Check sheet for the modelled part. Datum: model origin and axes. Units: mm. A direction names the side the tool comes from. Give positions to 0.01 mm unless a question says otherwise; leave off trailing zeros. Loops run counter-clockwise (first coordinate to the right, second up) from the corner with the lowest first, then second, coordinate; pieces in that order, holes last. Notation, with made-up numbers: (36, -29.5) - (74, -29.5) arc R19 cw to (74, -6.5) - close; hole circle Ø11 at (-24.5, 62). An arc over 180 degrees is marked (long way). Use one line per item in the form item = value.
from build123d import *

# Parameters (mm, degrees)
BOSS_EXTRUDE1_DEPTH      = 1.5
BOSS_EXTRUDE1_DEPTH_BACK = 5
SKETCH1_R                = 10.1
SKETCH1_R_2              = 8.6
SKETCH2_R                = 10.1
BOSS_EXTRUDE2_DEPTH      = 1.5
SKETCH3_R                = 1.75
CUT_EXTRUDE1_DEPTH       = 1.5


with BuildPart() as part:
    # Sketch1 → Boss-Extrude1 (new, two sides: drawn at the far end of the back side and taken through both)
    with BuildSketch(Plane.XY.offset(-BOSS_EXTRUDE1_DEPTH_BACK)):
        with Locations((-10.160617153, 18.12022925)):
            Circle(SKETCH1_R)
        with Locations((-10.160617153, 18.12022925)):
            Circle(SKETCH1_R_2, mode=Mode.SUBTRACT)
    extrude(amount=BOSS_EXTRUDE1_DEPTH + BOSS_EXTRUDE1_DEPTH_BACK)

    # Sketch2 → Boss-Extrude2 (add)
    with BuildSketch(Plane.XY.offset(1.5)):
        with Locations((-10.160617153, 18.12022925)):
            Circle(SKETCH2_R)
    extrude(amount=-BOSS_EXTRUDE2_DEPTH)

    # Sketch3 → Cut-Extrude1 (cut)
    with BuildSketch(Plane.XY.offset(1.5)):
        with Locations((-16.460617153, 18.12022925)):
            Circle(SKETCH3_R)
    extrude(amount=-CUT_EXTRUDE1_DEPTH, mode=Mode.SUBTRACT)


solid = part.part
Item 1: Access from +Z, -Z, +X, -X, +Y, -Y to the whole of each face (thin tool, end or side, straight path). Record for faces 1 (the face through (-10, 18, 0)), 2 (the face through (-2.7, 22.7, -5)).
Answer block:
face_1 = -Z
face_2 = -Z, +X, -X, +Y, -Y
Item 2: Section check C-C on x = -9. Record the boundary of the cut face in (y, z).
Answer block:
outline = (8.09, -5) - (9.6, -5) - (9.6, 0) - (26.64, 0) - (26.64, -5) - (28.15, -5) - (28.15, 1.5) - (8.09, 1.5) - close
Item 3: Gauge pin test, flat ends, axial feed: P1, Ø1, axis at y = 19, z = -0.5, coming from the +X side; P2, Ø1, axis at y = 16, z = -3, coming from the +X side; P3, Ø8.5, axis at x = -10, y = 15, coming from the -Z side. Record the tip position at first contact, or that the pin passes through.
Answer block:
P1 = -0.07
P2 = -0.19
P3 = 0
Item 4: Thickness scan on L1, parallel to X at y = 18.25, z = 0.25; L2, parallel to Z at x = -8.5, y = 9.75; L3, parallel to Y at x = -15.5, z = -2. Record the ranges inside material, lowest first.
Answer block:
L1 = -20.26 to -18.21, -14.72 to -0.06
L2 = 0 to 1.5
L3 = 9.55 to 11.38, 24.86 to 26.69
Item 5: Mould release check, pull along Y, two halves, no side actions. Record for faces 3 (the face through (-10, 18, 1.5)), 4 (the face through (-11.28, 26.647, -2.535)), 5 (the face through (-0.527, 21.154, -1.796)): released by +Y, released by -Y, zero draft, split by the parting line, or undercut.
Answer block:
face_3 = zero draft
face_4 = undercut
face_5 = split by the parting line
Item 6: Section check B-B on y = 17. Record the boundary of the cut face in (x, z), then the cut area to 3 significant figures.
Answer block:
outline = (-20.2, -5) - (-18.69, -5) - (-18.69, 0) - (-17.81, 0) - (-17.81, 1.5) - (-20.2, 1.5) - close; (-15.12, 0) - (-1.63, 0) - (-1.63, -5) - (-0.12, -5) - (-0.12, 1.5) - (-15.12, 1.5) - close
area = 41.2 mm2
Item 7: Section check D-D on z = 0.25. Record the boundary of the cut face in (x, y).
Answer block:
outline = circle Ø20.2 at (-10.16, 18.12); hole circle Ø3.5 at (-16.46, 18.12)
Item 8: Section check A-A on x = -17.75. Record the boundary of the cut face in (y, z), then the cut area to 3 significant figures.
Answer block:
outline = (11.46, -5) - (14.08, -5) - (14.08, 0) - (16.94, 0) - (16.94, 1.5) - (11.46, 1.5) - close; (19.3, 0) - (22.17, 0) - (22.17, -5) - (24.78, -5) - (24.78, 1.5) - (19.3, 1.5) - close
area = 42.6 mm2
